Autodesk Inventor part; units mm, degrees
ref_plane "YZ Plane" through (0, 0, 0) normal (1, 0, 0) x (0, 1, 0)
ref_plane "XZ Plane" through (0, 0, 0) normal (0, 1, 0) x (-1, 0, 0)
ref_plane "XY Plane" through (0, 0, 0) normal (0, 0, 1) x (1, 0, 0)
sketch "Sketch1" plane through (0, 0, 0) normal (0, 0, 1) x (1, 0, 0)
  line L0 (-75, -60) -> (75, -60)
  line L1 (75, -60) -> (75, 60)
  line L2 (75, 60) -> (-75, 60)
  line L3 (-75, 60) -> (-75, -60)
  line L4 (-75, -60) -> (75, 60) construction
  line L5 (75, -60) -> (-75, 60) construction
  point P0 (0, 0)
  dimension "d0" = 150
  dimension "d1" = 120
extrude "Extrusion1" add sketch "Sketch1" against normal blind 10
sketch "Sketch2" plane through (0, 0, 0) normal (0, 0, 1) x (1, 0, 0)
  line L0 (-71, -56) -> (71, -56)
  line L1 (71, -56) -> (71, 56)
  line L2 (71, 56) -> (-71, 56)
  line L3 (-71, 56) -> (-71, -56)
  line L4 (-71, -56) -> (71, 56) construction
  line L5 (71, -56) -> (-71, 56) construction
  line L6 (75, 60) -> (-75, 60)
  line L7 (-75, 60) -> (-75, -60)
  line L8 (-68, -53) -> (68, -53)
  line L9 (68, -53) -> (68, 53)
  line L10 (68, 53) -> (-68, 53)
  line L11 (-68, 53) -> (-68, -53)
  line L12 (-68, -53) -> (68, 53) construction
  line L13 (68, -53) -> (-68, 53) construction
  point P0 (0, 0)
  dimension "d4" = 4
  dimension "d5" = 4
  dimension "d6" = 3
  dimension "d7" = 3
extrude "Extrusion2" add sketch "Sketch2" along normal blind 4
properties part number "Pi Case Top V 01" material "ABS Plastic"
Design review of the part built by this model. Coordinates are the model's own, in mm. A direction names the side the tool comes from. Give positions to 0.01 mm unless a question says otherwise; leave off trailing zeros. Order: outer loops, then holes, each group sorted by start corner. A loop starts at its lowest first (then second) coordinate and runs counter-clockwise, first axis right, second up. Notation, with made-up numbers: (-4.75, -21.75) - (36.25, -21.75) arc R7 ccw to (36.25, -8.75) - close; hole circle Ø7 at (66.5, -32.5). An arc over 180 degrees is marked (long way). Use a Markdown table: item, result. Add a question column.
(1) Wall thickness on probe 1 along Y at (x, z) = (15.5, 1); probe 2 along X at (y, z) = (-25, 3.25); probe 3 along Z at (x, y) = (34, -23.5): over which ranges is each line inside the solid? List them lowest first. Write a range as [from, to].
(2) Clearance check with flat-ended pins moving along their axes: P1, Ø3, axis at y = 22, z = 3, coming from the +X side; P2, Ø2, axis at x = 27, y = -17, coming from the +Z side; P3, Ø1.2, axis at x = -23, z = 2, coming from the -Y side. State where each tip first meets the part, or that it passes through.
(3) Machinability: for faces 1 (the face through (-1, -56, 2)), 2 (the face through (1, 56, 2)), 3 (the face through (71, -1, 2)), 4 (the face through (-1, -53, 2)), 5 (the face through (-71, 1, 2)), which of the approach directions +Z, -Z, +X, -X, +Y, -Y give a long, thin tool a straight path to every point of the face, cutting with its end or side? Answer none if there is none.
(4) Mouldability with a two-part tool opening along X and no side actions: class faces 6 (the face through (1, 53, 2)), 7 (the face through (-1, -60, -5)), 8 (the face through (75, -1, -5)) as +X half, -X half, draft (parallel to the pull), parting line (faces both ways), or undercut.
(5) Add section A-A on y = 42.5. Give the boundary of the cut face in (x, z), then the cut area to 3 significant figures.
(6) Add section B-B on x = -63.5. Give the boundary of the cut face in (y, z).
Report:
| question | item | result |
|---|---|---|
| 1 | probe 1 | y = [-56, -53], [53, 56] |
| 1 | probe 2 | x = [-71, -68], [68, 71] |
| 1 | probe 3 | z = [-10, 0] |
| 2 | P1 | stops at x = 71 |
| 2 | P2 | stops at z = 0 |
| 2 | P3 | stops at y = -56 |
| 3 | face 1 | +Z, +X, -X, -Y |
| 3 | face 2 | +Z, +X, -X, +Y |
| 3 | face 3 | +Z, +X, +Y, -Y |
| 3 | face 4 | +Z |
| 3 | face 5 | +Z, -X, +Y, -Y |
| 4 | face 6 | undercut |
| 4 | face 7 | draft |
| 4 | face 8 | +X half |
| 5 | outline | (-75, -10) - (75, -10) - (75, 0) - (71, 0) - (71, 4) - (68, 4) - (68, 0) - (-68, 0) - (-68, 4) - (-71, 4) - (-71, 0) - (-75, 0) - close |
| 5 | area | 1,520 mm² |
| 6 | outline | (-60, -10) - (60, -10) - (60, 0) - (56, 0) - (56, 4) - (53, 4) - (53, 0) - (-53, 0) - (-53, 4) - (-56, 4) - (-56, 0) - (-60, 0) - close |
